Build history of the part. All positions in model axes, mm. Face numbers are marked on the shaded views. A direction names the side the tool comes from. Round coordinates to 2 decimals unless told otherwise and drop trailing zeros. Write each loop counter-clockwise with the first axis right and the second up, starting at its lowest first coordinate (ties: lowest second). Pieces come first, ordered by that corner, then holes. Notation, with made-up numbers: M 12,8 L 69,8 A25 ccw 69,23 Z; hole C 74.25,-30.75 d1. An arc over 180 degrees is marked long. Write item = value, one per line.
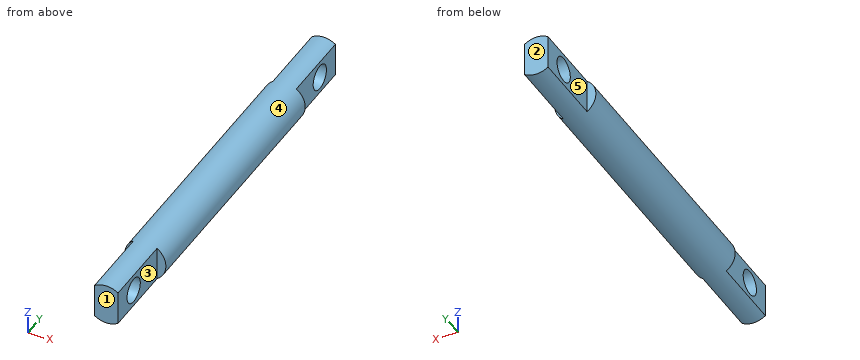
from build123d import *

# Parameters (mm, degrees)
SKETCH1_R                        = 7
BOSS_EXTRUDE1_DEPTH              = 139.254
SKETCH3_W                        = 3.842840079
SKETCH3_H                        = 19.362001934
SKETCH3_W_2                      = 3.621137766
CUT_EXTRUDE1_DEPTH               = 25
SKETCH4_W                        = 4.298001377
SKETCH4_H                        = 18.624672635
SKETCH4_W_2                      = 5.056472209
SKETCH4_H_2                      = 19.003908051
CUT_EXTRUDE2_DEPTH               = 25
TAP_DRILL_FOR_M10X1_5_TAP1_D     = 8.5
TAP_DRILL_FOR_M10X1_5_TAP1_DEPTH = 20
TAP_DRILL_FOR_M10X1_5_TAP1_TIP   = 2.553657631


with BuildPart() as part:
    # Sketch1 → Boss-Extrude1 (new body)
    with BuildSketch(Plane(origin=(0, 0, 0), x_dir=(1, 0, 0), z_dir=(0, 1, 0))):
        Circle(SKETCH1_R)
    extrude(amount=BOSS_EXTRUDE1_DEPTH)

    # Sketch3 → Cut-Extrude1 (cut)
    with BuildSketch(Plane.XZ):
        with Locations((5.92142004, -0.588495195)):
            Rectangle(SKETCH3_W, SKETCH3_H)
        with Locations((-5.810568883, -0.588495195)):
            Rectangle(SKETCH3_W_2, SKETCH3_H)
    extrude(amount=-CUT_EXTRUDE1_DEPTH, mode=Mode.SUBTRACT)

    # Sketch4 → Cut-Extrude2 (cut)
    with BuildSketch(Plane(origin=(0, 139.254, 0), x_dir=(1, 0, 0), z_dir=(0, 1, 0))):
        with Locations((-6.149000689, -0.400304049)):
            Rectangle(SKETCH4_W, SKETCH4_H)
        with Locations((6.528236105, -0.589921757)):
            Rectangle(SKETCH4_W_2, SKETCH4_H_2)
    extrude(amount=-CUT_EXTRUDE2_DEPTH, mode=Mode.SUBTRACT)

    # Tap Drill for M10x1.5 Tap1
    with Locations(Plane(origin=(4, 0, 0), x_dir=(0, 0, -1), z_dir=(1, 0, 0))):
        with Locations((0, 129.254), (0, 10)):
            Hole(TAP_DRILL_FOR_M10X1_5_TAP1_D / 2, depth=TAP_DRILL_FOR_M10X1_5_TAP1_DEPTH)
            with Locations((0, 0, -(TAP_DRILL_FOR_M10X1_5_TAP1_DEPTH + TAP_DRILL_FOR_M10X1_5_TAP1_TIP / 2))):  # 118° drill point
                Cone(0, TAP_DRILL_FOR_M10X1_5_TAP1_D / 2, TAP_DRILL_FOR_M10X1_5_TAP1_TIP, mode=Mode.SUBTRACT)


solid = part.part
1. Probe probe 1 along Y at (x, z) = (2, 0); probe 2 along X at (y, z) = (20.5, -3.25); probe 3 along X at (y, z) = (83.5, -0.5). List the from-to ranges inside material, lowest first.
Responses:
probe_1 = 0 to 5.75, 14.25 to 125, 133.5 to 139.25
probe_2 = -4 to 4
probe_3 = -6.98 to 6.98
2. Band-saw the part on A-A (z = 0). List the corners of the cut face in (x, y).
Responses:
outline = M -7,25 L -4,25 L -4,14.25 L 4,14.25 L 4,25 L 7,25 L 7,114.25 L 4,114.25 L 4,125 L -4,125 L -4,114.25 L -7,114.25 Z; M -4,0 L 4,0 L 4,5.75 L -4,5.75 Z; M -4,133.5 L 4,133.5 L 4,139.25 L -4,139.25 Z
3. Band-saw the part on B-B (y = 10). List the corners of the cut face in (x, z).
Responses:
outline = M -4,-5.74 A7 ccw 4,-5.74 L 4,-4.25 L -4,-4.25 Z; M -4,4.25 L 4,4.25 L 4,5.74 A7 ccw -4,5.74 Z
4. Flat gauge pins, fed straight in: pin 1 (1 mm diameter, centred on y = 108, z = 3.5, fed in from +X); pin 2 (8 mm diameter, centred on x = 4, z = -2.5, fed in from -Y); pin 3 (2 mm diameter, centred on x = -4, y = 101.5, fed in from -Z); pin 4 (5 mm diameter, centred on y = 10, z = 0, fed in from +X). Where does each tip first touch, or does it go through?
Responses:
pin_1 = 6.32
pin_2 = 0
pin_3 = -6.32
pin_4 = through
5. Tool access for the marked faces 4 and 5: list every direction of +Z, -Z, +X, -X, +Y, -Y with a clear straight run to the whole face (end or side of a thin tool).
Responses:
face_4 = +Y, -Y
face_5 = +Z, -Z, -X, +Y
6. Band-saw the part on D-D (x = -2). List the corners of the cut face in (y, z), plus the area to 3 significant figures.
Responses:
outline = M 0,-6.71 L 139.25,-6.71 L 139.25,6.71 L 0,6.71 Z; hole C 10,0 d8.5; hole C 129.25,0 d8.5
area = 1,750 mm²
7. Mould opens along Y. For the marked faces 1, 2 and 3 say: pulls with the +Y half, pulls with the -Y half, needs draft (parallel to the pull), parting line crosses it, or undercut.
Responses:
face_1 = pulls with the -Y half
face_2 = pulls with the +Y half
face_3 = needs draft
8. Band-saw the part on C-C (y = 83.5). List the corners of the cut face in (x, z), plus the area to 3 significant figures.
Responses:
outline = C 0,0 d14
area = 154 mm²
